Geometry check sheet. Reference: the model listing, model coordinates, mm. Face numbers are marked on the shaded views. A direction names the side the tool comes from. Give positions to 0.01 mm unless a question says otherwise; leave off trailing zeros. Order: outer loops, then holes, each group sorted by start corner. A loop starts at its lowest first (then second) coordinate and runs counter-clockwise, first axis right, second up. Notation, with made-up numbers: M 74,51.25 L 104,51.25 A32 ccw 104,87.25 Z; hole C 74,44.5 d1. An arc over 180 degrees is marked long. Answer as CSV lines item,"result".
from build123d import *

# Parameters (mm, degrees)
SKETCH_1_W          = 84
SKETCH_1_H          = 92
EXTRUDE_1_DEPTH     = 5
SKETCH_2_W          = 25
SKETCH_2_H          = 25
SKETCH_2_W_2        = 15
SKETCH_2_H_2        = 15
SKETCH_2_W_3        = 5.1
SKETCH_2_H_3        = 5
EXTRUDE_2_DEPTH     = 10
SKETCH_3_R          = 1.2
CUT_EXTRUDE_1_DEPTH = 10


with BuildPart() as part:
    # 草图1 → 凸台-拉伸1 (new body)
    with BuildSketch(Plane(origin=(0, 0, 0), x_dir=(1, 0, 0), z_dir=(0, 1, 0))):
        Rectangle(SKETCH_1_W, SKETCH_1_H)
    extrude(amount=EXTRUDE_1_DEPTH)

    # 草图2 → 凸台-拉伸2 (add)
    # profile 1 of 2: a face of its own
    with BuildSketch(Plane.XZ):
        Rectangle(SKETCH_2_W, SKETCH_2_H)
        Rectangle(SKETCH_2_W_2, SKETCH_2_H_2, mode=Mode.SUBTRACT)
    # profile 2 of 2: a face of its own
    with BuildSketch(Plane.XZ):
        Rectangle(SKETCH_2_W_3, SKETCH_2_H_3)
    extrude(amount=EXTRUDE_2_DEPTH)

    # 草图3 → 切除-拉伸1 (cut)
    with BuildSketch(Plane(origin=(0, 5, 0), x_dir=(1, 0, 0), z_dir=(0, 1, 0))):
        with Locations(Location((-37, -14, 0), (0, 0, 270))):
            Circle(SKETCH_3_R)
        with Locations(Location((5, -14, 0), (0, 0, 270))):
            Circle(SKETCH_3_R)
        with Locations(Location((-37, -41, 0), (0, 0, 270))):
            Circle(SKETCH_3_R)
        with Locations(Location((5, -41, 0), (0, 0, 270))):
            Circle(SKETCH_3_R)
        with Locations(Location((37, -9, 0), (0, 0, 270))):
            Circle(SKETCH_3_R)
        with Locations(Location((-37, -9, 0), (0, 0, 270))):
            Circle(SKETCH_3_R)
        with Locations(Location((-37, 41, 0), (0, 0, 270))):
            Circle(SKETCH_3_R)
        with Locations(Location((37, 41, 0), (0, 0, 270))):
            Circle(SKETCH_3_R)
    extrude(amount=-CUT_EXTRUDE_1_DEPTH, mode=Mode.SUBTRACT)


solid = part.part
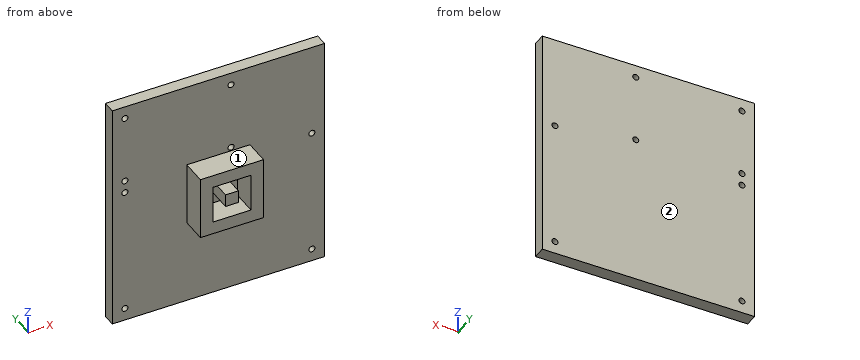
(1) Section check C-C on x = -37. Enter the section's corners in (y, z).
The answers:
outline,"M 0,-46 L 5,-46 L 5,-42.2 L 0,-42.2 Z; M 0,-39.8 L 5,-39.8 L 5,7.8 L 0,7.8 Z; M 0,10.2 L 5,10.2 L 5,12.8 L 0,12.8 Z; M 0,15.2 L 5,15.2 L 5,39.8 L 0,39.8 Z; M 0,42.2 L 5,42.2 L 5,46 L 0,46 Z"
(2) Section check B-B on x = 37. Enter the section's corners in (y, z).
The answers:
outline,"M 0,-46 L 5,-46 L 5,-42.2 L 0,-42.2 Z; M 0,-39.8 L 5,-39.8 L 5,7.8 L 0,7.8 Z; M 0,10.2 L 5,10.2 L 5,46 L 0,46 Z"
(3) Section check D-D on z = 41. Enter the section's corners in (x, y).
The answers:
outline,"M -42,0 L -38.2,0 L -38.2,5 L -42,5 Z; M -35.8,0 L 3.8,0 L 3.8,5 L -35.8,5 Z; M 6.2,0 L 42,0 L 42,5 L 6.2,5 Z"
(4) Gauge pin test, flat ends, axial feed: P1, Ø5, axis at y = -5, z = 3.5, coming from the +X side; P2, Ø1.5, axis at y = -5.5, z = -0.5, coming from the -X side; P3, Ø1, axis at x = -21.5, z = -20.5, coming from the -Y side. Record the tip position at first contact, or that the pin passes through.
The answers:
P1,"stops at x = 12.5"
P2,"stops at x = -12.5"
P3,"stops at y = 0"
(5) Tool access check on the marked faces 1 and 2. Record the directions out of +Z, -Z, +X, -X, +Y, -Y that give a thin tool (end or side, any length) a straight path to the whole face; none if there is none.
The answers:
face 1,"+Z, +X, -X, -Y"
face 2,"+Z, -Z, +X, -X, +Y"
(6) Section check A-A on z = 9. Enter the section's corners in (x, y), then the cut area to 3 significant figures.
The answers:
outline,"M -42,0 L -38.2,0 L -38.2,5 L -42,5 Z; M -35.8,0 L -12.5,0 L -12.5,-10 L 12.5,-10 L 12.5,0 L 35.8,0 L 35.8,5 L -35.8,5 Z; M 38.2,0 L 42,0 L 42,5 L 38.2,5 Z"
area,"646 mm2"
(7) Material ranges on line 1 (Z direction, x = -2, y = -7.75); line 2 (X direction, y = -7, z = -6.5), recorded low to high.
The answers:
line 1,"z = -12.5 to -7.5, -2.5 to 2.5, 7.5 to 12.5"
line 2,"x = -12.5 to -7.5, 7.5 to 12.5"
